Design review of the part built by this model. Coordinates are the model's own, in mm. Coordinates: 2 decimals unless noted, no trailing zeros. Write each loop counter-clockwise with the first axis right and the second up, starting at its lowest first coordinate (ties: lowest second). Pieces come first, ordered by that corner, then holes.
Q1. Mouldability with a two-part tool opening along Z and no side actions: class faces 1 (the flat face through (0, 15, -61)), 2 (the flat face through (0, 45, -100)), 3 (the flat face through (-38.05, 7.4, -57.07)) as pulls with the +Z half, pulls with the -Z half, needs draft (parallel to the pull), parting line crosses it, or undercut.
Q2. Take a section at A-A (y = 29.5). Give the boundary of the cut face in (x, z), and give its area (3 significant figures).
Q3. Insertion check: pin 1 (1.5 mm diameter, centred on x = 10.5, y = 22.5, fed in from -Z); pin 2 (3 mm diameter, centred on x = -40, z = -4.5, fed in from +Y); pin 3 (8 mm diameter, centred on x = -27, y = 30, fed in from -Z). Each pin has a flat end and moves straight along its axis. Give the tip position at first contact, or say it passes through.
Q4. For probe 1 along Z at (x, y) = (12, 36); probe 2 along Y at (x, z) = (-30, -38); probe 3 along X at (y, z) = (-3.5, -106), list the stretches that pass through material, from the lowest coordinate up.
Q5. Take a section at B-B (y = 9.5). Give the boundary of the cut face in (x, z), and give its area (3 significant figures).
Autodesk Inventor part; units mm, degrees
ref_plane "Work Plane1" through (47.6941, 7.5, -9.7355) normal (0, 1, 0) x (1, 0, 0)
ref_plane "YZ Plane" through (0, 0, 0) normal (1, 0, 0) x (0, 1, 0)
ref_plane "XZ Plane" through (0, 0, 0) normal (0, 1, 0) x (-1, 0, 0)
sketch "Sketch1" plane through (0, 0, 0) normal (0, 1, 0) x (-1, 0, 0)
  arc A0 (-48.9898, -10) -> (48.9898, -10) centre (0, 0) ccw construction
  line L0 (0, 0) -> (0, -100) construction
  arc A1 (29.3939, -106) -> (-29.3939, -106) centre (0, -100) ccw construction
  line L1 (48.9898, -10) -> (29.3939, -106)
  line L2 (-48.9898, -10) -> (-29.3939, -106)
  arc A2 (48.9898, -10) -> (-48.9898, -10) centre (0, 0) ccw
  arc A3 (-29.3939, -106) -> (29.3939, -106) centre (0, -100) ccw
  dimension "d0" = 100
  dimension "d1" = 100
  dimension "d2" = 60
extrude "Extrusion1" add sketch "Sketch1" along normal mid plane 30 draft -10
ref_plane "Work Plane1" through (47.6941, 7.5, -9.7355) normal (0, 1, 0) x (1, 0, 0)
sketch "Sketch2" plane through (0, 15, 0) normal (0, 1, 0) x (1, 0, 0)
  line L0 (-46.3983, 9.471) -> (-26.8024, 105.471)
  circle A0 centre (0, 0) radius 47.3551
extrude "Extrusion2" add sketch "Sketch2" along normal blind 30 draft -30
sketch "Sketch3" plane through (0, 15, 0) normal (0, 1, 0) x (1, 0, 0)
  arc A0 (26.8024, 105.471) -> (-26.8024, 105.471) centre (0, 100) ccw
  circle A1 centre (0, 100) radius 27.3551
  point P0 (0, 0)
  point P1 (-26.8024, 105.471)
  dimension "d7" = 54.7102
extrude "Extrusion3" add sketch "Sketch3" along normal blind 30 draft -30
fillet "Fillet1" radius 5 6 edges at (-30.0346, 45, 0) (-9.8318, 45, -97.9931) (0, -15, -127.3551) (-36.6004, -15, -57.471) (0, -15, 47.3551) (36.6004, -15, -57.471)
properties part number "LE-1.1"
Response:
1. face 1: undercut
1. face 2: needs draft
1. face 3: pulls with the -Z half
2. outline: circle Ø77.97 at (0, 0); (-18.6, -103.8) arc R18.98 ccw to (18.6, -103.8) arc R18.98 ccw (long way) to start
2. area: 5,910 mm2
3. pin 1: stops at z = -121.1
3. pin 2: stops at y = 29.9
3. pin 3: stops at z = -32.28
4. probe 1: z = -109.38 to -90.62, -33.12 to 33.12
4. probe 2: y = -15 to 15
4. probe 3: x = -28.76 to 28.76
5. outline: (-47.35, -9.66) - (-27.75, -105.66) arc R28.32 ccw to (27.75, -105.66) - (47.35, -9.66) arc R48.32 ccw (long way) to start
5. area: 12,700 mm2
